Autodesk Inventor part; units mm, degrees
ref_plane "YZ Plane" through (0, 0, 0) normal (1, 0, 0) x (0, 1, 0)
ref_plane "XZ Plane" through (0, 0, 0) normal (0, 1, 0) x (-1, 0, 0)
ref_plane "XY Plane" through (0, 0, 0) normal (0, 0, 1) x (1, 0, 0)
sketch "Sketch1" plane through (0, 0, 0) normal (0, 0, 1) x (1, 0, 0)
  line L0 (-135, 115) -> (135, 115)
  line L1 (135, 115) -> (135, -115)
  line L2 (135, -115) -> (-135, -115)
  line L3 (-135, -115) -> (-135, 115)
  line L4 (-110, 92.5) -> (110, 92.5)
  line L5 (110, 92.5) -> (110, -92.5)
  line L6 (110, -92.5) -> (-110, -92.5)
  line L7 (-110, -92.5) -> (-110, 92.5)
  point P0 (0, 0)
  point P1 (0, 115)
  point P2 (0, 92.5)
  point P3 (-110, 0)
  point P4 (-135, 0)
  dimension "d0" = 270
  dimension "d1" = 230
  dimension "d2" = 220
  dimension "d3" = 185
extrude "Extrusion1" add sketch "Sketch1" against normal blind 15 contours L4 L5 L6 L7
extrude "Extrusion2" add sketch "Sketch1" along normal blind 10 contours L0 L1 L2 L3 | L4 L5 L6 L7
chamfer "Chamfer1" distance 5 angle 45 4 edges at (0, 92.5, -15) (110, 0, -15) (0, -92.5, -15) (-110, 0, -15)
sketch "Sketch2" plane through (0, 0, 10) normal (0, 0, 1) x (1, 0, 0)
  line L0 (125, -107.5) -> (125, 107.5)
  line L1 (-125, 107.5) -> (-125, -107.5)
  line L2 (125, 107.5) -> (-125, 107.5)
  line L3 (-125, -107.5) -> (125, -107.5)
  line L4 (0, 107.5) -> (0, -107.5)
  line L5 (-135, -115) -> (135, -115)
  line L6 (135, -115) -> (135, 115)
  line L7 (135, 115) -> (-135, 115)
  line L8 (-135, 115) -> (-135, -115)
  point P0 (0, 0)
  point P1 (-117.5, 100)
  point P2 (-39.1667, 100)
  point P3 (39.1667, 100)
  point P4 (117.5, 100)
  point P5 (-117.5, 33.3333)
  point P6 (-117.5, -33.3333)
  point P7 (-117.5, -100)
  point P8 (-200.4459, 0)
  point P9 (-39.1667, -100)
  point P10 (39.1667, -100)
  point P11 (117.5, -100)
  point P12 (117.5, 33.3333)
  point P13 (117.5, -33.3333)
  dimension "d19" = 250
  dimension "d22" = 7.5
  dimension "d23" = 7.5
  dimension "d24" = 78.3333
  dimension "d25" = 215
  dimension "d26" = 66.6667
hole "Hole1" at (117.5, -33.3333, 10) at (117.5, 33.3333, 10) at (117.5, -100, 10) at (39.1667, -100, 10) at (-39.1667, -100, 10) at (-117.5, -100, 10) at (-117.5, -33.3333, 10) at (-117.5, 33.3333, 10) at (117.5, 100, 10) at (39.1667, 100, 10) at (-39.1667, 100, 10) at (-117.5, 100, 10) direction (0, 0, -1) diameter 8.376 depth 27.3 tip angle 118
chamfer "Chamfer2" distance 2 angle 45 4 edges at (0, 115, 10) (-135, 0, 10) (135, 0, 10) (0, -115, 10)
sketch "Sketch3" plane through (0, 0, 10) normal (0, 0, 1) x (1, 0, 0)
  circle A0 centre (-117.5, 100) radius 4.188
  circle A1 centre (39.1667, 100) radius 4.188
  circle A2 centre (-117.5, 33.3333) radius 4.188
  circle A3 centre (-117.5, -100) radius 4.188
  circle A4 centre (39.1667, -100) radius 4.188
  circle A5 centre (117.5, 33.3333) radius 4.188
  circle A6 centre (117.5, -33.3333) radius 4.188
  circle A7 centre (117.5, -100) radius 4.188
  circle A8 centre (-39.1667, -100) radius 4.188
  circle A9 centre (-117.5, -33.3333) radius 4.188
  circle A10 centre (117.5, 100) radius 4.188
  circle A11 centre (-39.1667, 100) radius 4.188
  line L0 (133, -113) -> (-133, -113)
  line L1 (133, 113) -> (133, -113)
  line L2 (-133, 113) -> (133, 113)
  line L3 (-133, -113) -> (-133, 113)
  circle A12 centre (-117.5, 100) radius 8
  circle A13 centre (-39.167, 100) radius 8
  circle A14 centre (39.166, 100) radius 8
  circle A15 centre (117.499, 100) radius 8
  circle A16 centre (-117.5, 33.333) radius 8
  circle A17 centre (-117.5, -33.334) radius 8
  circle A18 centre (-117.5, -100.001) radius 8
  circle A19 centre (-39.167, -100.001) radius 8
  circle A20 centre (39.166, -100.001) radius 8
  circle A21 centre (117.499, -100.001) radius 8
  circle A22 centre (117.499, 33.333) radius 8
  circle A23 centre (117.499, -33.334) radius 8
  point P0 (0, 0)
  dimension "d39" = 16
  dimension "d42" = 78.333
  dimension "d49" = 66.667
  dimension "d56" = 78.333
  dimension "d63" = 66.667
extrude "Extrusion3" cut sketch "Sketch3" against normal blind 10 contours A0 | A1 | A2 | A3 | A4 | A5 | A6 | A7 | A8 | A9 | A10 | A11 | A12 | A13 | A14 | A15 | A16 | A17 | A18 | A19 | A20 | A21 | A22 | A23
properties part number "Cover of base" material "Steel, Alloy"
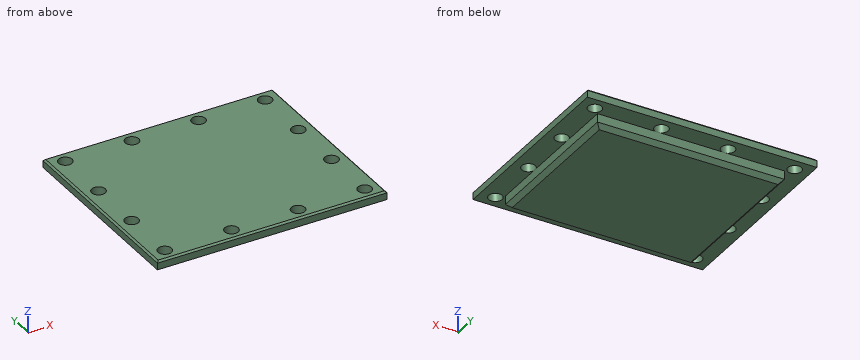
Check sheet for the modelled part. Datum: model origin and axes. Units: mm. Give positions to 0.01 mm unless a question says otherwise; leave off trailing zeros. Order: outer loops, then holes, each group sorted by start corner. A loop starts at its lowest first (then second) coordinate and runs counter-clockwise, first axis right, second up. Notation, with made-up numbers: (7, 4.25) -> (50, 4.25) arc R15 cw to (50, 26.25) -> close; hole circle Ø9 at (76.5, 65). An arc over 180 degrees is marked (long way). Return JSON: item names as keys, results as strings.
1. Cross-section at A-A, the plane y = 100. Record the cut outline in (x, z).
From the geometry:
{"outline": "(-135, 0) -> (-125.5, 0) -> (-125.5, 10) -> (-133, 10) -> (-135, 8) -> close; (-109.5, 0) -> (-47.17, 0) -> (-47.17, 10) -> (-109.5, 10) -> close; (-31.17, 0) -> (31.17, 0) -> (31.17, 10) -> (-31.17, 10) -> close; (47.17, 0) -> (109.5, 0) -> (109.5, 10) -> (47.17, 10) -> close; (125.5, 0) -> (135, 0) -> (135, 8) -> (133, 10) -> (125.5, 10) -> close"}
2. Cross-section at C-C, the plane x = 67.5. Record the cut outline in (y, z).
From the geometry:
{"outline": "(-115, 0) -> (-92.5, 0) -> (-92.5, -10) -> (-87.5, -15) -> (87.5, -15) -> (92.5, -10) -> (92.5, 0) -> (115, 0) -> (115, 8) -> (113, 10) -> (-113, 10) -> (-115, 8) -> close"}
3. Go/stop test with flat-tipped pins: P1, Ø9.5, axis at x = 117.499, y = 33.333, coming from the -Z side; P2, Ø5, axis at x = -41, z = -7.5, coming from the -Y side; P3, Ø10, axis at y = -44.5, z = -10, coming from the +X side; P4, Ø6, axis at y = 4.5, z = -4.5, coming from the -X side. Record where each tip stops, or that it passes through.
From the geometry:
{"P1": "through", "P2": "y = -92.5", "P3": "x = 110", "P4": "x = -110"}
4. Cross-section at D-D, the plane y = 75. Record the cut outline in (x, z).
From the geometry:
{"outline": "(-135, 0) -> (-110, 0) -> (-110, -10) -> (-105, -15) -> (105, -15) -> (110, -10) -> (110, 0) -> (135, 0) -> (135, 8) -> (133, 10) -> (-133, 10) -> (-135, 8) -> close"}
5. Material ranges on probe 1 along Y at (x, z) = (117, 0.25); probe 2 along Y at (x, z) = (-117.5, 7); probe 3 along Y at (x, z) = (-35.5, 2), recorded low to high. Write a range as [from, to].
From the geometry:
{"probe 1": "[-115, -107.99], [-92.02, -41.32], [-25.35, 25.35], [41.32, 92.02], [107.98, 115]", "probe 2": "[-115, -108], [-92, -41.33], [-25.33, 25.33], [41.33, 92], [108, 115]", "probe 3": "[-115, -107.11], [-92.89, 92.89], [107.11, 115]"}
6. Cross-section at B-B, the plane x = -117.5. Record the cut outline in (y, z), plus the area to 3 significant figures.
From the geometry:
{"outline": "(-115, 0) -> (-108, 0) -> (-108, 10) -> (-113, 10) -> (-115, 8) -> close; (-92, 0) -> (-41.33, 0) -> (-41.33, 10) -> (-92, 10) -> close; (-25.33, 0) -> (25.33, 0) -> (25.33, 10) -> (-25.33, 10) -> close; (41.33, 0) -> (92, 0) -> (92, 10) -> (41.33, 10) -> close; (108, 0) -> (115, 0) -> (115, 8) -> (113, 10) -> (108, 10) -> close", "area": "1,660 mm^2"}
